The figure shows three views and two pictorial views of one solid part (mm, origin at its lowest corner). Answer the questions. Coordinates: 2 decimals unless noted, no trailing zeros. Loops run counter-clockwise (first coordinate to the right, second up) from the corner with the lowest first, then second, coordinate; pieces in that order, holes last. Notation, with made-up numbers: (4, 27) - (22, 27) arc R26 ccw to (22, 49) - close; hole circle Ø5 at (55, 39.5). An arc over 180 degrees is marked (long way). Write each question's results on one line, items separated by ' | '. Start each with the question number.
Item 1: For a pull along Z with two mould halves and no side action, classify the marked faces 1, 2 and 3 as +Z half, -Z half, draft (parallel to the pull), parting line (faces both ways), or undercut.
Item 2: Consider probe 1 along Z at (x, y) = (73, 9) (1 decimal); probe 2 along Z at (x, y) = (20, 7) (1 decimal); probe 3 along X at (y, z) = (8.75, 5.5). Determine where each line is inside the solid, lowest interval first. Write a range as [from, to].
Item 3: Section B-B, the plane z = 46 is taken. Write down the section's boundary in (x, y), plus the area to 3 significant figures.
Item 4: Section C-C, the plane x = 80 is taken. Write down the section's boundary in (y, z).
Item 5: This flat-tipped pin is pushed along its axis until it touches: pin 1 Ø15.5 at (x, z) = (65.44, 23.73) entering from +Y. Where does it stop, or does it pass through?
Item 6: Section A-A, the plane y = 3 is taken. Write down the section's boundary in (x, z) (1 decimal).
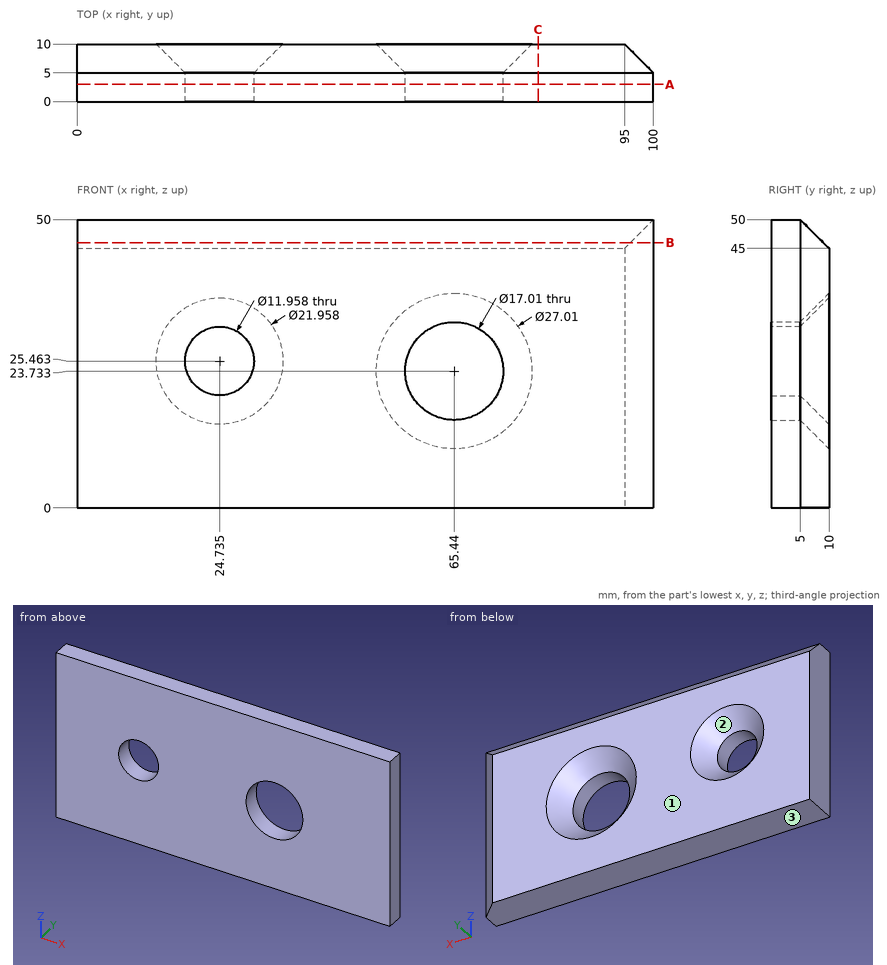
Answer key:
1) face 1: draft | face 2: undercut | face 3: -Z half
2) probe 1: z = [0, 13.8], [33.7, 46] | probe 2: z = [0, 19], [31.9, 48] | probe 3: x = [0, 96.25]
3) outline: (0, 0) - (100, 0) - (100, 5) - (96, 9) - (0, 9) - close | area: 892 mm^2
4) outline: (0, 0) - (10, 0) - (10, 45) - (5, 50) - (0, 50) - close
5) pin 1: passes through
6) outline: (0, 0) - (100, 0) - (100, 50) - (0, 50) - close; hole circle Ø12 at (24.7, 25.5); hole circle Ø17 at (65.4, 23.7)
